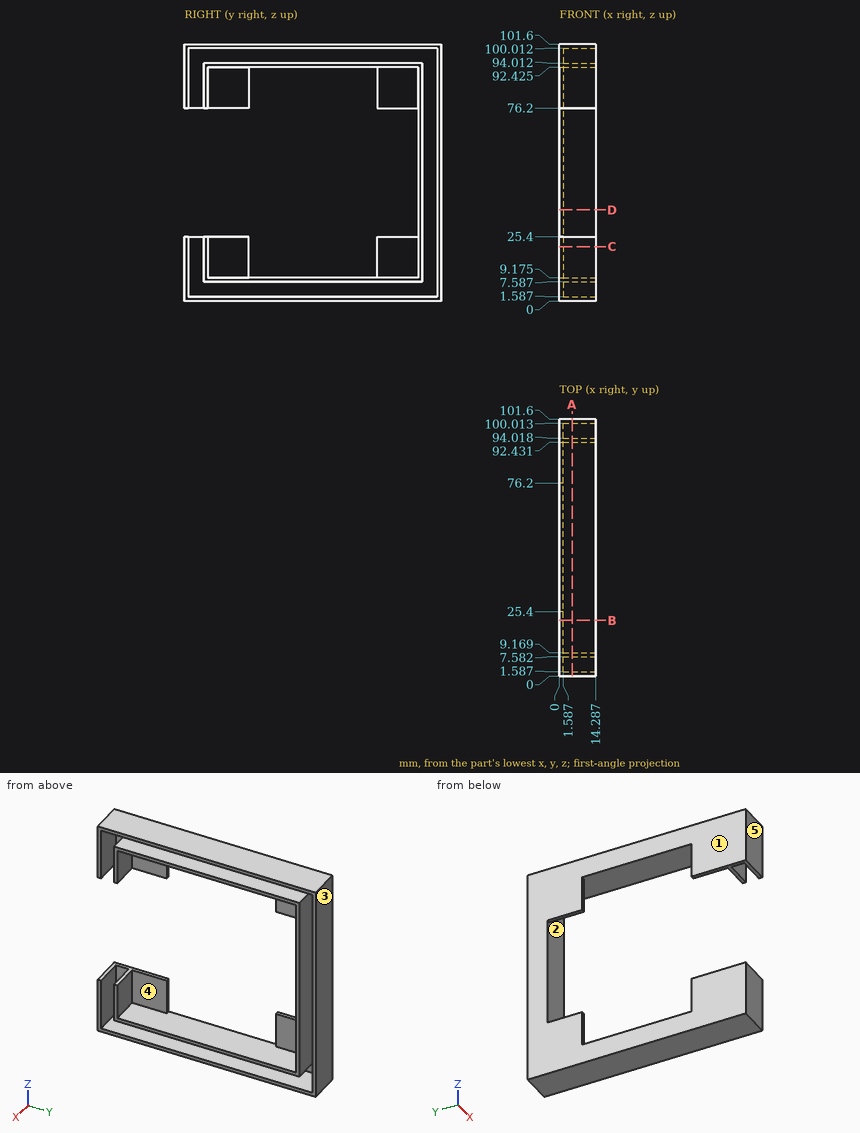
Answer from the drawing. Dimensions are ordinates in mm from the lowest x, y and z of the part. A direction names the side the tool comes from. Round coordinates to 2 decimals unless told otherwise and drop trailing zeros. Order: outer loops, then holes, each group sorted by start corner. A loop starts at its lowest first (then second) coordinate and runs counter-clockwise, first axis right, second up. Notation, with made-up numbers: (15, 62.25) - (62, 62.25) arc R23 ccw to (62, 95.25) - close; hole circle Ø7 at (8.25, 57.25). An arc over 180 degrees is marked (long way). Put each result on its own line as item: value. Start each with the question number.
(1) Find section A-A (x = 5). Give the vertices of the cut face in (y, z) (1 decimal).
(2) Find section B-B (y = 22). Give the vertices of the cut face in (x, z) (1 decimal).
(3) Determine the mould class of the marked faces 1, 2 and 3 for opening direction Y: released by +Y, released by -Y, zero draft, split by the parting line, or undercut.
(4) Straight lines are drawn through the part: probe 1 along Z at (x, y) = (11, 91.5) (1 decimal); probe 2 along Y at (x, z) = (5.25, 81.5); probe 3 along Y at (x, z) = (1.5, 24.5). For each, find the intervals that lie inside material, in ascending order. Write a range as from..to.
(5) Find section D-D (z = 36). Give the vertices of the cut face in (x, y).
(6) For the marked faces 4 and 5, determine the directions among +Z, -Z, +X, -X, +Y, -Y from which every point of the face is accessible in a straight line to the end or side of a thin tool.
(7) Given P1, Ø18, axis at y = 81.5, z = 80.5, coming from the +X side, flat-ended and moving along its own axis, determine where the tip first touches the part or whether it passes through.
(8) Find section C-C (z = 21.5). Give the vertices of the cut face in (x, y).
Reply:
1. outline: (0, 0) - (101.6, 0) - (101.6, 101.6) - (0, 101.6) - (0, 76.2) - (1.6, 76.2) - (1.6, 100) - (100, 100) - (100, 1.6) - (1.6, 1.6) - (1.6, 25.4) - (0, 25.4) - close; (7.6, 7.6) - (94, 7.6) - (94, 94) - (7.6, 94) - (7.6, 76.2) - (9.2, 76.2) - (9.2, 92.4) - (92.4, 92.4) - (92.4, 9.2) - (9.2, 9.2) - (9.2, 25.4) - (7.6, 25.4) - close
2. outline: (0, 0) - (14.3, 0) - (14.3, 1.6) - (1.6, 1.6) - (1.6, 7.6) - (14.3, 7.6) - (14.3, 9.2) - (1.6, 9.2) - (1.6, 25.4) - (0, 25.4) - close; (0, 76.2) - (1.6, 76.2) - (1.6, 92.4) - (14.3, 92.4) - (14.3, 94) - (1.6, 94) - (1.6, 100) - (14.3, 100) - (14.3, 101.6) - (0, 101.6) - close
3. face 1: zero draft
3. face 2: undercut
3. face 3: released by +Y
4. probe 1: 0..1.6, 7.6..9.2, 92.4..94, 100..101.6
4. probe 2: 0..1.59, 7.58..9.17, 92.43..94.02, 100.01..101.6
4. probe 3: 0..25.4, 76.2..101.6
5. outline: (0, 92.43) - (14.29, 92.43) - (14.29, 94.02) - (1.59, 94.02) - (1.59, 100.01) - (14.29, 100.01) - (14.29, 101.6) - (0, 101.6) - close
6. face 4: +X
6. face 5: +Z, -Z, +X, -X, -Y
7. P1: x = 1.59
8. outline: (0, 0) - (14.29, 0) - (14.29, 1.59) - (1.59, 1.59) - (1.59, 7.58) - (14.29, 7.58) - (14.29, 9.17) - (1.59, 9.17) - (1.59, 25.4) - (0, 25.4) - close; (0, 76.2) - (1.59, 76.2) - (1.59, 92.43) - (14.29, 92.43) - (14.29, 94.02) - (1.59, 94.02) - (1.59, 100.01) - (14.29, 100.01) - (14.29, 101.6) - (0, 101.6) - close
